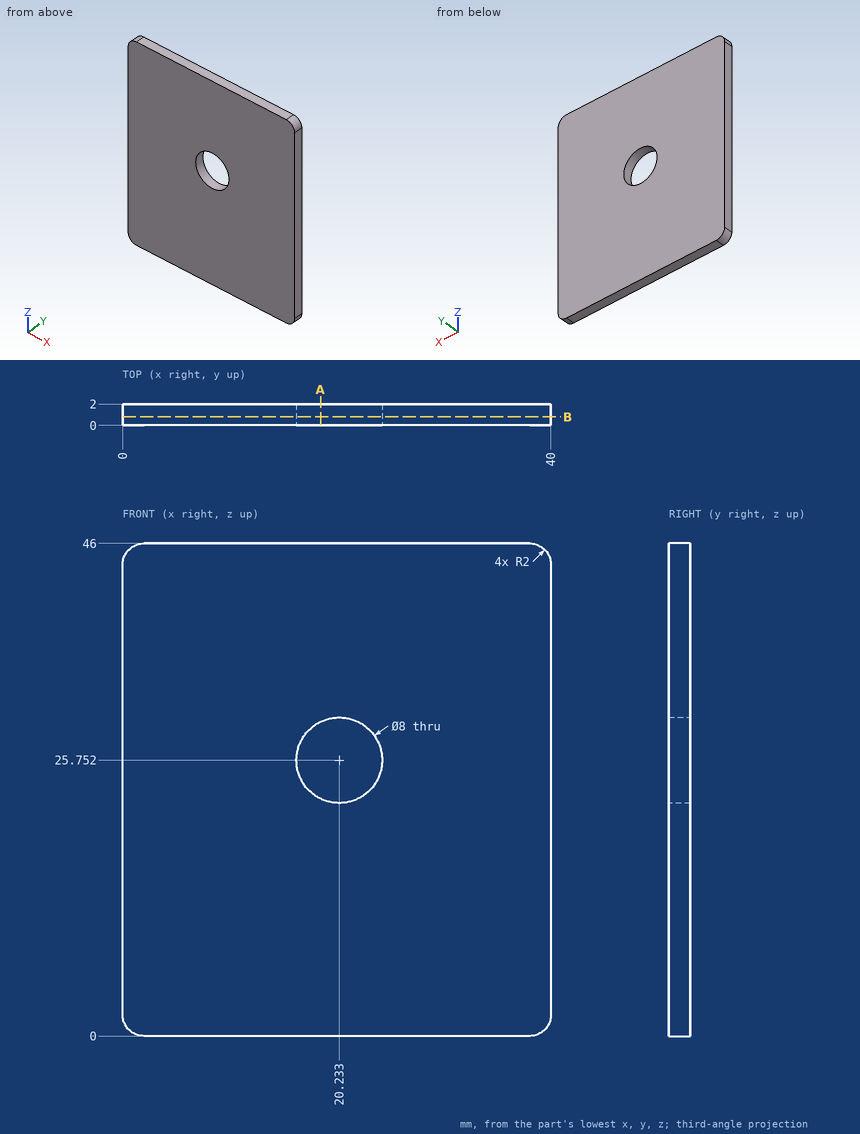
Source: three-view drawing plus pictorial views. Frame: mm from the lowest corner of the part. Round coordinates to 2 decimals unless told otherwise and drop trailing zeros. Loops run counter-clockwise (first coordinate to the right, second up) from the corner with the lowest first, then second, coordinate; pieces in that order, holes last. Notation, with made-up numbers: (5.5, -16) -> (19.5, -16) arc R26 ccw to (19.5, 20) -> close; hole circle Ø3 at (69.25, 26). An arc over 180 degrees is marked (long way). Use one line per item in the form item = value.
Item 1: Material intervals for probe 1 along Z at (x, y) = (22, 0.9); probe 2 along Z at (x, y) = (19.5, 1.1); probe 3 along X at (y, z) = (0.8, 28) (1 decimal), sorted ascending.
Evaluation:
probe_1 = 0 to 22.16, 29.34 to 46
probe_2 = 0 to 21.82, 29.68 to 46
probe_3 = 0 to 16.9, 23.5 to 40
Item 2: Cut plane B-B on y = 0.8. Output: boundary loops of the cut face in (x, z), then the cut area to 3 significant figures.
Evaluation:
outline = (0, 2) arc R2 ccw to (2, 0) -> (38, 0) arc R2 ccw to (40, 2) -> (40, 44) arc R2 ccw to (38, 46) -> (2, 46) arc R2 ccw to (0, 44) -> close; hole circle Ø8 at (20.23, 25.75)
area = 1,790 mm2
Item 3: Cut plane A-A on x = 18.5. Output: boundary loops of the cut face in (y, z).
Evaluation:
outline = (0, 0) -> (2, 0) -> (2, 22.15) -> (0, 22.15) -> close; (0, 29.36) -> (2, 29.36) -> (2, 46) -> (0, 46) -> close
